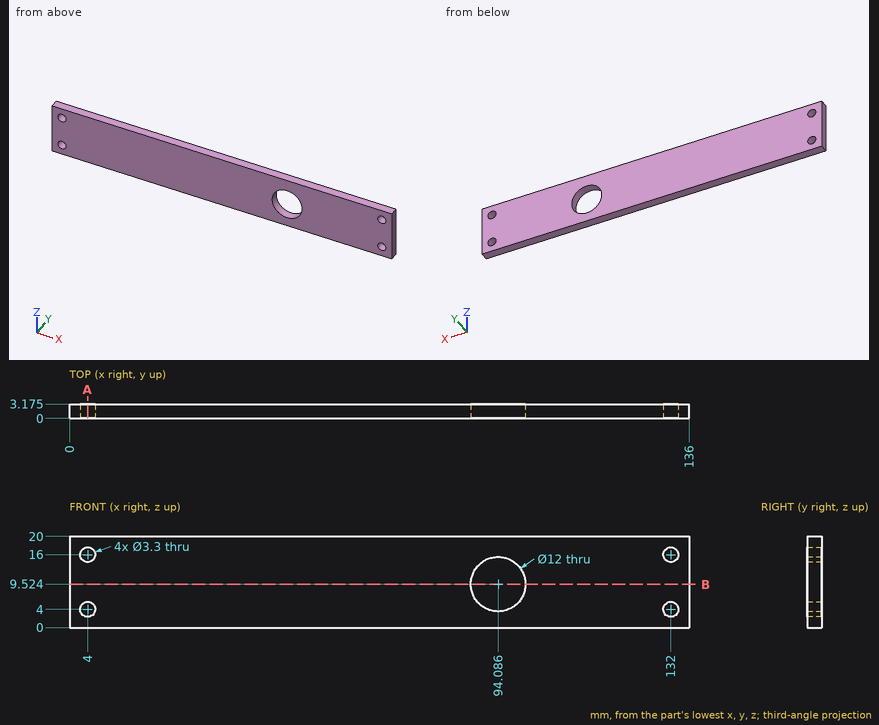
Design review of the part shown in the three views and the two pictorial views. Dimensions are in mm from the part's minimum x, y and z. Coordinates: 2 decimals unless noted, no trailing zeros. Write each loop counter-clockwise with the first axis right and the second up, starting at its lowest first coordinate (ties: lowest second). Pieces come first, ordered by that corner, then holes.
1) Clearance check with a flat-ended pin moving along its axis: pin 1 Ø2.5 at (x, z) = (4, 4) entering from -Y. State where the tip first meets the part, or that it passes through.
2) We need section B-B on z = 9.5. State the section outline as (x, y) points (1 decimal).
3) To check wall thickness, follow probe 1 along Z at (x, y) = (132, 1.3); probe 2 along X at (y, z) = (2.1, 16); probe 3 along X at (y, z) = (1.85, 9). State the ranges of each line that lie inside material, in increasing order.
4) We need section A-A on x = 4. Count the separate pieces of the cut face and the enclosed holes in it.
Answer list:
1. pin 1: passes through
2. outline: (0, 0) - (88.1, 0) - (88.1, 3.2) - (0, 3.2) - close; (100.1, 0) - (136, 0) - (136, 3.2) - (100.1, 3.2) - close
3. probe 1: z = 0 to 2.35, 5.65 to 14.35, 17.65 to 20
3. probe 2: x = 0 to 2.35, 5.65 to 130.35, 133.65 to 136
3. probe 3: x = 0 to 88.11, 100.06 to 136
4. separate pieces: 3
4. enclosed holes: 0
